Read the model definition and answer for the solid it produces. Units are mm, in the model's axes. A direction names the side the tool comes from. Give positions to 0.01 mm unless a question says otherwise; leave off trailing zeros. Order: outer loops, then holes, each group sorted by start corner. A loop starts at its lowest first (then second) coordinate and runs counter-clockwise, first axis right, second up.
```python
from build123d import *

# Parameters (mm, degrees)
BOSS_EXTRUDE1_DEPTH = 3.302
FILLET1_R           = 0.508
SKETCH3_W           = 6.35
SKETCH3_H           = 0.762
BOSS_EXTRUDE2_DEPTH = 11.43
SKETCH4_W           = 6.35
SKETCH4_H           = 0.762
BOSS_EXTRUDE3_DEPTH = 11.43
CHAMFER1_SIZE       = 1.016


with BuildPart() as part:
    # Sketch1 → Base-Revolve (revolve)
    with BuildSketch(Plane(origin=(0, 0, 0), x_dir=(1, 0, 0), z_dir=(0, 1, 0))):
        Polygon((0, -17.78), (6.858, -17.78), (7.747, -9.652), (6.35, -9.652), (6.35, -8.382), (7.747, -8.382), (7.747, 0), (6.35, 0), (6.35, 6.096), (4.699, 6.096), (4.699, 25.146), (0, 25.146), align=None)
    revolve(axis=Axis((0, 0, 0), (0, 0, -1)))

    # Sketch2 → Boss-Extrude1 (add)
    with BuildSketch(Plane(origin=(0, 0, -4.826), x_dir=(-1, 0, 0), z_dir=(0, 0, -1))):
        Polygon((-6.394250991, -7.45995949), (3.263388934, -9.267563542), (9.657639925, -1.807604052), (6.394250991, 7.45995949), (-3.263388934, 9.267563542), (-9.657639925, 1.807604052), align=None)
    extrude(amount=-BOSS_EXTRUDE1_DEPTH)

    # Fillet1
    fillet1_edges = [part.edges().sort_by_distance(p)[0] for p in [
        (-6.858, 0, 17.78),
    ]]
    fillet(fillet1_edges, radius=FILLET1_R)

    # Sketch3 → Boss-Extrude2 (add)
    with BuildSketch(Plane(origin=(0, 0, -25.146), x_dir=(-1, 0, 0), z_dir=(0, 0, -1))):
        with Locations((0, 2.921)):
            Rectangle(SKETCH3_W, SKETCH3_H)
    extrude(amount=BOSS_EXTRUDE2_DEPTH)

    # Sketch4 → Boss-Extrude3 (add)
    with BuildSketch(Plane(origin=(-0.217554927, 1.748253857, -6.096), x_dir=(-1, 0, 0), z_dir=(0, 0, -1))):
        with Locations((-0.217554927, 3.712746143)):
            Rectangle(SKETCH4_W, SKETCH4_H)
    extrude(amount=BOSS_EXTRUDE3_DEPTH)

    # Chamfer1
    chamfer1_edges = [part.edges().sort_by_distance(p)[0] for p in [
        (3.175, 5.461, -17.526),
        (-3.175, 5.461, -17.526),
        (-3.175, 2.921, -36.576),
        (3.175, 2.921, -36.576),
    ]]
    chamfer(chamfer1_edges, length=CHAMFER1_SIZE)


solid = part.part
```
1) A tool of negligible diameter and unlimited length cuts with its end or side. For faces 5 (the face through (-0.61, -4.66, -15.75)), 6 (the face through (0, 5.08, -12)), 7 (the face through (0, 3.302, -31)), 8 (the face through (-6, -3, 9.652)), 9 (the face through (6.416, 5.59, -3.198)), from which of +Z, -Z, +X, -X, +Y, -Y can it reach the whole face along a straight path? Write none if from no direction.
Final values:
face 5: -Z
face 6: -Z, +X, -X
face 7: -Z, +X, -X, +Y
face 8: none
face 9: +Z, -Z, +X, +Y
2) Given pin 1 (4 mm diameter, centred on y = -3.5, z = -10, fed in from -X); pin 2 (0.6 mm diameter, centred on y = 3, z = -31.5, fed in from -X) (3 decimals); pin 3 (0.6 mm diameter, centred on x = 0.5, y = 5.5, fed in from -Z), each flat-ended and moving along its own axis, determine where each tip first touches the part or whether it passes through.
Final values:
pin 1: stops at x = -4.45
pin 2: stops at x = -3.175
pin 3: stops at z = -17.53
3) The part is cut by section C-C on z = 7.5. Determine the outline of the cut face in (x, y), and give its area (3 significant figures).
Final values:
outline: circle Ø15.49 at (0, 0)
area: 189 mm2
4) Consider L1, parallel to Z at x = -8, y = -1.5; L2, parallel to Z at x = 3.75, y = 1.5; L3, parallel to Y at x = -0.25, z = -5.5. Determine where each line is inside the solid, lowest interval first.
Final values:
L1: z = -4.83 to -1.52
L2: z = -25.15 to 17.78
L3: y = -6.35 to 6.35
5) For a pull along Z with two mould halves and no side action, classify faces 1 (the face through (0, 0, 17.78)), 2 (the face through (-1.38, 6.2, -0.77)), 3 (the face through (-8.05, 2.76, -3.2)), 4 (the face through (-1.38, 6.2, 9.01)) as released by +Z, released by -Z, zero draft, split by the parting line, or undercut.
Final values:
face 1: released by +Z
face 2: undercut
face 3: zero draft
face 4: undercut
6) The part is cut by section A-A on z = -20. Determine the outline of the cut face in (x, y).
Final values:
outline: circle Ø9.4 at (0, 0)
7) The part is cut by section D-D on x = 8.5. Determine the outline of the cut face in (y, z).
Final values:
outline: (-1.48, -4.83) - (3.16, -4.83) - (3.16, -1.52) - (-1.48, -1.52) - close
